Build history of the part. All positions in model axes, mm. A direction names the side the tool comes from. Give positions to 0.01 mm unless a question says otherwise; leave off trailing zeros. Loops run counter-clockwise (first coordinate to the right, second up) from the corner with the lowest first, then second, coordinate; pieces in that order, holes last. Notation, with made-up numbers: (55, -27.75) -> (92, -27.75) arc R10 ccw to (92, -17.75) -> close; hole circle Ø1 at (41, 76.5). An arc over 180 degrees is marked (long way). Answer in a Markdown table with one row per item. Add a question column.
Autodesk Inventor part; units mm, degrees
ref_plane "YZ Plane" through (0, 0, 0) normal (1, 0, 0) x (0, 1, 0)
ref_plane "XZ Plane" through (0, 0, 0) normal (0, 1, 0) x (-1, 0, 0)
ref_plane "XY Plane" through (0, 0, 0) normal (0, 0, 1) x (1, 0, 0)
sketch "Эскиз1" plane through (0, 0, 0) normal (0, 0, 1) x (1, 0, 0)
  line L0 (-25, -109) -> (25, -109)
  line L1 (25, -109) -> (25, 109)
  line L2 (25, 109) -> (-25, 109)
  line L3 (-25, 109) -> (-25, -109)
  line L4 (-25, -109) -> (25, 109) construction
  line L5 (25, -109) -> (-25, 109) construction
  line L6 (0, 0) -> (0, 129.6236) construction
  line L7 (0, 0) -> (116.4638, 0) construction
  line L8 (-25, 109) -> (-10, 109)
  line L9 (-10, 109) -> (-10, 115)
  line L10 (-10, 115) -> (-25, 115)
  line L11 (-25, 115) -> (-25, 109)
  line L12 (25, 109) -> (10, 109)
  line L13 (10, 109) -> (10, 115)
  line L14 (10, 115) -> (25, 115)
  line L15 (25, 115) -> (25, 109)
  line L16 (-25, -109) -> (-10, -109)
  line L17 (-10, -109) -> (-10, -115)
  line L18 (-10, -115) -> (-25, -115)
  line L19 (-25, -115) -> (-25, -109)
  line L20 (25, -109) -> (10, -109)
  line L21 (10, -109) -> (10, -115)
  line L22 (10, -115) -> (25, -115)
  line L23 (25, -115) -> (25, -109)
  dimension "d0" = 50
  dimension "d1" = 15
  dimension "d2" = 6
  dimension "d3" = 230
extrude "Выдавливание1" add sketch "Эскиз1" along normal mid plane 6
sketch "Эскиз2" plane through (0, 0, 3) normal (0, 0, 1) x (1, 0, 0)
  point P0 (0, 0)
sketch "Эскиз3" plane through (0, 0, 3) normal (0, 0, 1) x (1, 0, 0)
  line L0 (-41.4458, -60) -> (-5, -60)
  line L1 (-5, -60) -> (-5, 50)
  line L2 (-5, 50) -> (-41.4458, 50)
  line L3 (-41.4458, 50) -> (-41.4458, -60)
  line L4 (-25, -115) -> (-10, -115)
  line L5 (-25, 115) -> (-25, -115)
  line L6 (-25, 50) -> (-19, 50)
  line L7 (-19, 50) -> (-19, 44)
  line L8 (-19, 44) -> (-25, 44)
  line L9 (-25, 44) -> (-25, 50)
  point P0 (0, 0)
  dimension "d8" = 20
  dimension "d12" = 6
  dimension "d13" = 6
  dimension "d17" = 50
  dimension "d18" = 60
extrude "Выдавливание2" cut sketch "Эскиз3" against normal through all contours L3 L2 L5 L0 | L5 L8 L7 L2 L1 L0
fillet "Сопряжение1" radius 10 3 edges at (-5, -60, 0) (-5, 50, 0) (-25, -60, 0)
fillet "Сопряжение2" radius 2 3 edges at (-19, 44, 0) (-25, 44, 0) (-19, 50, 0)
properties part number "Планка боковая"
(1) 3-axis set-ups, long thin cutter, end or side, ignore diameter. For faces 4 (the cylindrical face through (-8.01, 47.15, -0.04)), 5 (the flat face through (-5, -6, 0)), 6 (the flat face through (-25, -92, 0)), 7 (the flat face through (-10, 112, 0)), 8 (the flat face through (10, -112, 0)): which of +Z, -Z, +X, -X, +Y, -Y reach the whole face in a straight line?
(2) Saw through at B-B, the plane y = -16.5. List the corners of the cut face in (x, z), then the cut area to 3 significant figures.
(3) Flat gauge pin, fed straight in: pin 1 Ø3 at (y, z) = (14.5, -1) entering from -X. Where does the tip first touch, or does it go through?
(4) Saw through at C-C, the plane x = 4. List the corners of the cut face in (y, z).
(5) Wall check: line 1 along Y through (x, z) = (-14.5, -1.75); line 2 along X through (y, z) = (11, 0.4); line 3 along Y through (x, z) = (-4, -1.95). Give the ranges that are in metal, low to high. Write a range as from..to.
(6) Two-plate mould, pull along X, no slides. Class faces 1 (the flat face through (17, -115, 0)), 2 (the flat face through (-25, 81, 0)), 3 (the flat face through (0, 109, 0)): released by +X, released by -X, zero draft, split by the parting line, or undercut.
Worked answers:
| question | item | result |
|---|---|---|
| 1 | face 4 | +Z, -Z |
| 1 | face 5 | +Z, -Z, -X |
| 1 | face 6 | +Z, -Z, -X, +Y, -Y |
| 1 | face 7 | +Z, -Z, +Y |
| 1 | face 8 | +Z, -Z, -Y |
| 2 | outline | (-5, -3) -> (25, -3) -> (25, 3) -> (-5, 3) -> close |
| 2 | area | 180 mm^2 |
| 3 | pin 1 | x = -5 |
| 4 | outline | (-109, -3) -> (109, -3) -> (109, 3) -> (-109, 3) -> close |
| 5 | line 1 | -115..-59.99, 49.99..115 |
| 5 | line 2 | -5..25 |
| 5 | line 3 | -109..109 |
| 6 | face 1 | zero draft |
| 6 | face 2 | released by -X |
| 6 | face 3 | undercut |
